Check sheet for the drawn part. Datum: minimum x, y, z corner. Units: mm. Coordinates: 2 decimals unless noted, no trailing zeros. Order: outer loops, then holes, each group sorted by start corner. A loop starts at its lowest first (then second) coordinate and runs counter-clockwise, first axis right, second up. Notation, with made-up numbers: M 30.5,29.5 L 86.5,29.5 A27 ccw 86.5,52.5 Z; hole C 14,86 d2. An arc over 180 degrees is marked long. Return JSON: item names as keys, results as strings. Group by question number.
Q1. Section check D-D, the plane z = 465. Enter the section's corners in (x, y).
Q2. Section check B-B, the plane z = 62. Enter the section's corners in (x, y), then the cut area to 3 significant figures.
Q3. Go/stop test with flat-tipped pins: pin 1 Ø25 at (y, z) = (388, 58) entering from +X; pin 2 Ø25 at (x, y) = (991, 379) entering from -Z; pin 3 Ø25 at (x, y) = (978.5, 540.5) entering from +Z. Record where each tip stops, or that it passes through.
Q4. Thickness scan on probe 1 along Z at (x, y) = (68.5, 367); probe 2 along X at (y, z) = (387.5, 719.5); probe 3 along Y at (x, z) = (143, 470.5). Record the ranges inside material, lowest first.
Q5. Section check A-A, the plane y = 227.5. Enter the section's corners in (x, z).
Q6. Section check C-C, the plane x = 862. Enter the section's corners in (y, z).
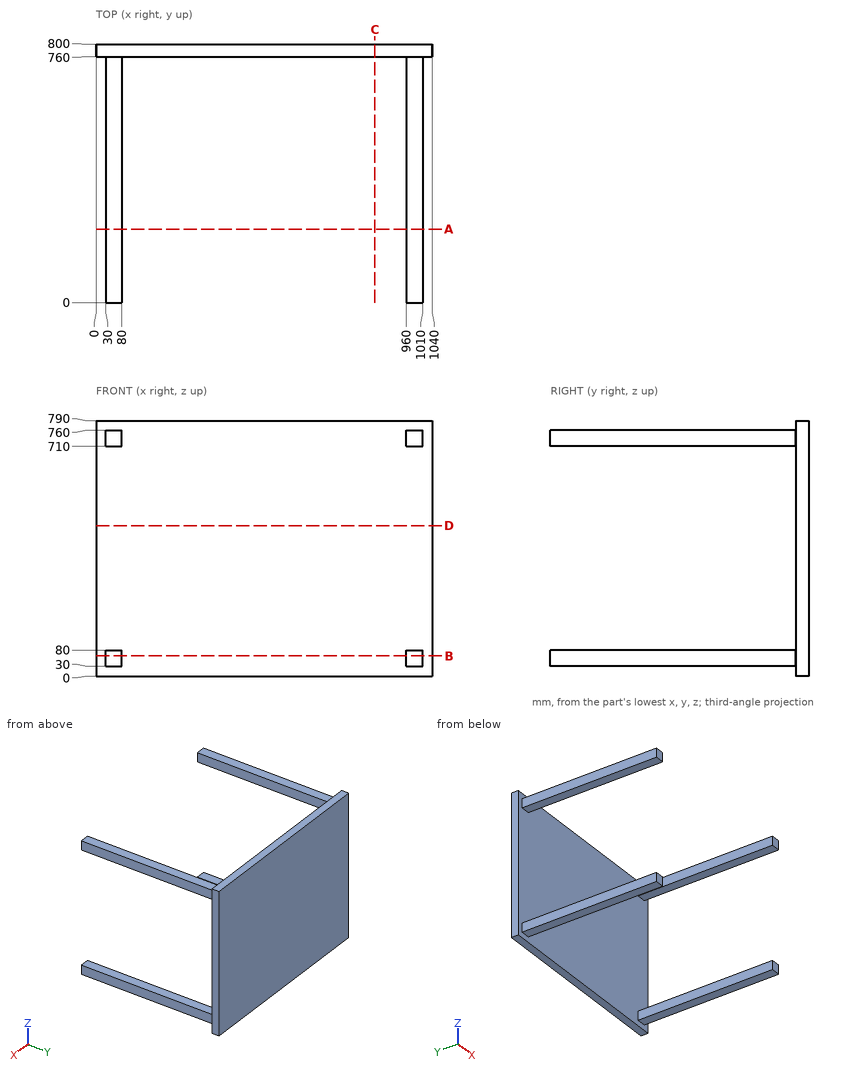
Numbers:
{
 "1": {"outline": "M 0,760 L 1040,760 L 1040,800 L 0,800 Z"},
 "2": {"outline": "M 0,760 L 30,760 L 30,0 L 80,0 L 80,760 L 960,760 L 960,0 L 1010,0 L 1010,760 L 1040,760 L 1040,800 L 0,800 Z", "area": "118,000 mm2"},
 "3": {"pin 1": "stops at x = 1010", "pin 2": "stops at z = 30", "pin 3": "stops at z = 760"},
 "4": {"probe 1": "z = 30 to 80, 710 to 760", "probe 2": "x = 30 to 80, 960 to 1010", "probe 3": "y = 760 to 800"},
 "5": {"outline": "M 30,30 L 80,30 L 80,80 L 30,80 Z; M 30,710 L 80,710 L 80,760 L 30,760 Z; M 960,30 L 1010,30 L 1010,80 L 960,80 Z; M 960,710 L 1010,710 L 1010,760 L 960,760 Z"},
 "6": {"outline": "M 760,0 L 800,0 L 800,790 L 760,790 Z"}
}
